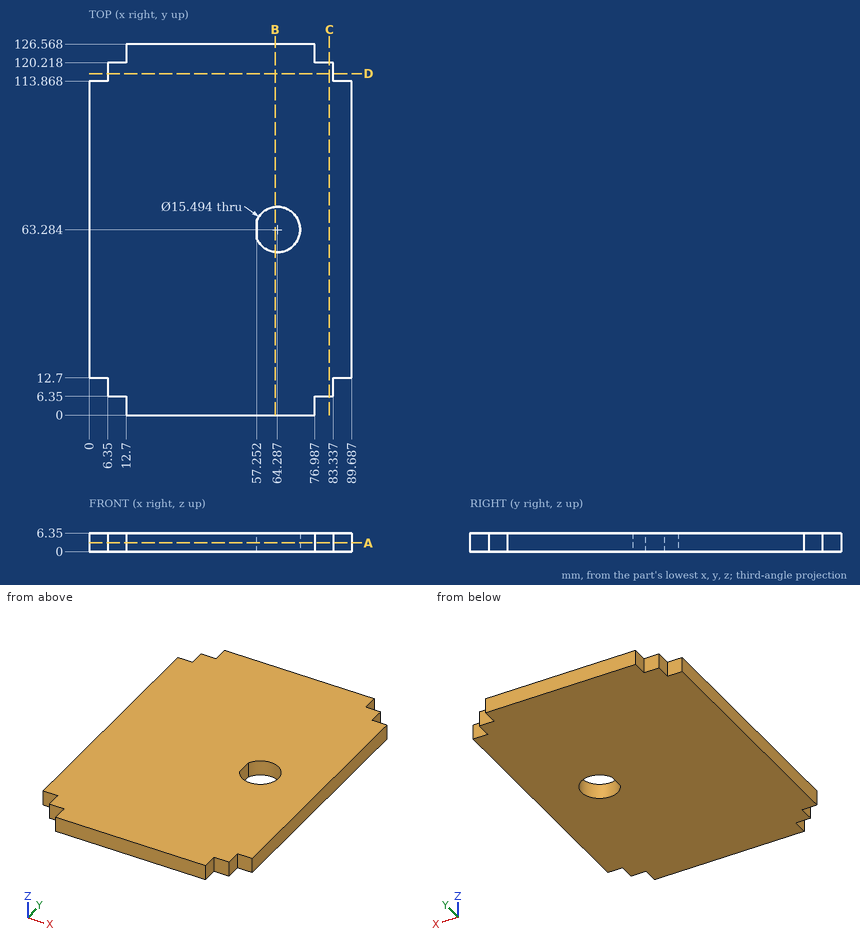
Here's the drawing with two shaded views (mm, measured from the low corner). I have some questions. Give positions to 0.01 mm unless a question says otherwise; leave off trailing zeros. Write each loop counter-clockwise with the first axis right and the second up, starting at its lowest first coordinate (ties: lowest second). Pieces come first, ordered by that corner, then holes. Notation, with made-up numbers: (-19, 9.25) - (-12, 9.25) arc R22 cw to (-12, 30.25) - close; hole circle Ø8 at (-24, 26). An arc over 180 degrees is marked (long way). Write item = value, one per line. Start each with the question number.
1. For pin 1 (3 mm diameter, centred on y = 117.5, z = 4.5, fed in from +X); pin 2 (3 mm diameter, centred on y = 123.5, z = 3.5, fed in from -X); pin 3 (3 mm diameter, centred on x = 9.5, z = 2.5, fed in from +Y), each with a flat end and sliding along its axis, tell me the tip position at first contact or that it passes through.
2. Imagine slicing it at C-C (x = 82). Please give me the cut outline in (y, z), and give its area (3 significant figures).
3. Imagine slicing it at D-D (y = 116.5). Please give me the cut outline in (x, z).
4. Imagine slicing it at B-B (x = 63.5). Please give me the cut outline in (y, z).
5. Please list where these lines run through material, in increasing order: line 1 (Y direction, x = 64, z = 6) (1 decimal); line 2 (X direction, y = 116.5, z = 5.75); line 3 (X direction, y = 66, z = 0.5).
6. Imagine slicing it at A-A (z = 3). Please give me the cut outline in (x, y), and give its area (3 significant figures).
Worked answers:
q1.pin_1 = 83.34
q1.pin_2 = 12.7
q1.pin_3 = 120.22
q2.outline = (6.35, 0) - (120.22, 0) - (120.22, 6.35) - (6.35, 6.35) - close
q2.area = 723 mm2
q3.outline = (6.35, 0) - (83.34, 0) - (83.34, 6.35) - (6.35, 6.35) - close
q4.outline = (0, 0) - (55.58, 0) - (55.58, 6.35) - (0, 6.35) - close; (70.99, 0) - (126.57, 0) - (126.57, 6.35) - (70.99, 6.35) - close
q5.line_1 = 0 to 55.5, 71 to 126.6
q5.line_2 = 6.35 to 83.34
q5.line_3 = 0 to 57.25, 71.54 to 89.69
q6.outline = (0, 12.7) - (6.35, 12.7) - (6.35, 6.35) - (12.7, 6.35) - (12.7, 0) - (76.99, 0) - (76.99, 6.35) - (83.34, 6.35) - (83.34, 12.7) - (89.69, 12.7) - (89.69, 113.87) - (83.34, 113.87) - (83.34, 120.22) - (76.99, 120.22) - (76.99, 126.57) - (12.7, 126.57) - (12.7, 120.22) - (6.35, 120.22) - (6.35, 113.87) - (0, 113.87) - close; hole (57.25, 60.04) arc R7.75 ccw (long way) to (57.25, 66.53) - close
q6.area = 10,700 mm2
